from build123d import *

# Parameters (mm, degrees)
F1_DEPTH       = 76.2
F4_D           = 38.1
F4_CBORE_D     = 50.8
F4_CBORE_DEPTH = 12.7
F5_D           = 38.1
F5_CBORE_D     = 50.8
F5_CBORE_DEPTH = 12.7


with BuildPart() as f1:
    # F0 (on Front) → F1 (new body)
    with BuildSketch(Plane.XZ):
        with BuildLine():
            Line((0, 76.2), (0, 0))
            Line((0, 0), (177.8, 0))
            Line((177.8, 0), (177.8, 28.575))
            Line((177.8, 28.575), (82.55, 28.575))
            Line((82.55, 28.575), (82.55, 76.2))
            ThreePointArc((82.55, 76.2), (41.275, 117.475), (0, 76.2))
        make_face()
    extrude(amount=F1_DEPTH)

    # F4 (through all)
    with Locations(Plane.XZ.offset(76.2)):
        with Locations((41.275, 76.2)):
            CounterBoreHole(F4_D / 2, F4_CBORE_D / 2, F4_CBORE_DEPTH)

    # F5 (through all)
    with Locations(Plane.XY.offset(28.575)):
        with Locations((139.7, -38.1)):
            CounterBoreHole(F5_D / 2, F5_CBORE_D / 2, F5_CBORE_DEPTH)


solid = f1.part
Work out the finished part from the listing and answer in its coordinate system (mm). A direction names the side the tool comes from. Coordinates: 2 decimals unless noted, no trailing zeros. Loops run counter-clockwise (first coordinate to the right, second up) from the corner with the lowest first, then second, coordinate; pieces in that order, holes last. Notation, with made-up numbers: M 22,-38 L 27,-38 A25 cw 27,-4 Z; hole C 36.5,29.25 d9. An arc over 180 degrees is marked long. Answer in a Markdown table with one row per item. Add a question column.
1. Consider L1, parallel to X at y = -68, z = 76; L2, parallel to X at y = -38, z = 24; L3, parallel to Y at x = 139, z = 26. Determine where each line is inside the solid, lowest interval first.
2. A tool of negligible diameter and unlimited length cuts with its end or side. For faces 5 (the cylindrical face through (54.93, -69.939, 97.617)), 6 (the flat face through (68, -76.2, 47)), 7 (the flat face through (143, -19, 15.875)), 8 (the flat face through (110, -38, 28.575)), from which of +Z, -Z, +X, -X, +Y, -Y can it reach the whole face along a straight path? Write none if from no direction.
3. Find section B-B, the plane y = -6. Write down the section's boundary in (x, z) (3 decimals), then the cut area to 3 significant figures.
4. Find section A-A, the plane y = -38.1. Write down the section's boundary in (x, z) (3 decimals).
5. The mould has two halves that part along Y. Classify faces 1 (the flat face through (82.55, -38, 52)), 2 (the cylindrical face through (158.73, -37.26, 7.83)), 3 (the flat face through (68, 0, 47)), 4 (the cylindrical face through (163.927, -30.471, 22.314)): pulls with the +Y half, pulls with the -Y half, needs draft (parallel to the pull), parting line crosses it, or undercut.
6. Find section C-C, the plane x = 139.7. Write down the section's boundary in (y, z) (3 decimals), then the cut area to 3 significant figures.
7. Flat-ended cylindrical pins translate along their axes: P1, Ø3, axis at y = -18.5, z = 73, coming from the +X side; P2, Ø1, axis at y = -33, z = 98.5, coming from the -X side; P3, Ø4, axis at x = 121, y = -36.5, coming from the +Z side (3 decimals); P4, Ø23, axis at x = 41.275, z = 76.2, coming from the +Y side. Find the tip coordinate at first contact, or state that the pin passes through.
8. Find section D-D, the plane z = 70. Write down the section's boundary in (x, y).
Reported:
| question | item | result |
|---|---|---|
| 1 | L1 | x = 0 to 15.88, 66.67 to 82.55 |
| 1 | L2 | x = 0 to 114.3, 165.1 to 177.8 |
| 1 | L3 | y = -76.2 to -63.49, -12.71 to 0 |
| 2 | face 5 | -Y |
| 2 | face 6 | +Z, -Z, +X, -X, -Y |
| 2 | face 7 | +Z |
| 2 | face 8 | +Z, +X, +Y, -Y |
| 3 | outline | M 0,0 L 177.8,0 L 177.8,28.575 L 82.55,28.575 L 82.55,76.2 A41.275 ccw 0,76.2 Z; hole C 41.275,76.2 d38.1 |
| 3 | area | 10,500 mm^2 |
| 4 | outline | M 0,0 L 120.65,0 L 120.65,15.875 L 114.3,15.875 L 114.3,28.575 L 82.55,28.575 L 82.55,76.2 A41.275 ccw 0,76.2 Z; M 158.75,0 L 177.8,0 L 177.8,28.575 L 165.1,28.575 L 165.1,15.875 L 158.75,15.875 Z; hole C 41.275,76.2 d38.1 |
| 5 | face 1 | needs draft |
| 5 | face 2 | undercut |
| 5 | face 3 | pulls with the +Y half |
| 5 | face 4 | undercut |
| 6 | outline | M -76.2,0 L -57.15,0 L -57.15,15.875 L -63.5,15.875 L -63.5,28.575 L -76.2,28.575 Z; M -19.05,0 L 0,0 L 0,28.575 L -12.7,28.575 L -12.7,15.875 L -19.05,15.875 Z |
| 6 | area | 927 mm^2 |
| 7 | P1 | stops at x = 82.55 |
| 7 | P2 | stops at x = 6.23 |
| 7 | P3 | stops at z = 15.875 |
| 7 | P4 | passes through |
| 8 | outline | M 0,-76.2 L 16.64,-76.2 L 16.64,-63.5 L 23.26,-63.5 L 23.26,0 L 0,0 Z; M 59.29,-63.5 L 65.91,-63.5 L 65.91,-76.2 L 82.55,-76.2 L 82.55,0 L 59.29,0 Z |
